Design review of the part built by this model. Coordinates are the model's own, in mm. A direction names the side the tool comes from. Give positions to 0.01 mm unless a question says otherwise; leave off trailing zeros. Order: outer loops, then holes, each group sorted by start corner. A loop starts at its lowest first (then second) coordinate and runs counter-clockwise, first axis right, second up. Notation, with made-up numbers: (44, 7.5) -> (63, 7.5) arc R19 ccw to (63, 19.5) -> close; hole circle Ø1 at (89.25, -9). An arc over 180 degrees is marked (long way). One line per item, written item: value. Start each with the question number.
1) Tool access review of faces 5 (the face through (6, 0, -5)), 6 (the face through (4.88, -1.08, -19.68)), 7 (the face through (2.6, -0.1, -11.4)): name each direction out of +Z, -Z, +X, -X, +Y, -Y from which nothing blocks a thin tool from reaching the whole face with its end or side.
2) Consider section C-C (x = 0). State the section outline as (y, z) points, plus the area to 3 significant figures.
3) Consider section B-B (z = 0). State the section outline as (x, y) points.
4) The part is to be moulded in two halves that separate along Z. For faces 1 (the face through (-4, -3, 0)), 2 (the face through (3, 1, -24)), 3 (the face through (5, -3, 0)), 4 (the face through (4, 6, -7)), say which applies: released by +Z, released by -Z, zero draft, split by the parting line, or undercut.
5) Wall thickness on line 1 along X through (y, z) = (4.25, -8.5); line 2 along X through (y, z) = (-0.25, 6); line 3 along Z through (x, y) = (5.35, 0): over which ranges is each line inside the solid? List them lowest first. Write a range as from..to.
6) Consider section D-D (z = -5). State the section outline as (x, y) points, plus the area to 3 significant figures.
7) Consider section A-A (y = 0). State how many separate pieces and enclosed holes the cut face has, plus the area to 3 significant figures.
8) For pin 1 (3.5 mm diameter, centred on y = 0, z = 0, fed in from +X); pin 2 (1 mm diameter, centred on x = -4.5, y = -3, fed in from +Z), all flat-tipped, find the tip position at first contact; note any pin that passes through.
from build123d import *

# Parameters (mm, degrees)
CUT_EXTRUDE1_DEPTH           = 13
CUT_EXTRUDE1_DEPTH_BACK      = 13
CUT_EXTRUDE2_DEPTH           = 13
CUT_EXTRUDE2_DEPTH_BACK      = 13
CUT_EXTRUDE3_DEPTH           = 13
CUT_EXTRUDE3_DEPTH_BACK      = 13
SKETCH5_W                    = 16.2
SKETCH5_H                    = 3
CUT_REVOLVE3_ANGLE           = 90
CUT_REVOLVE3_OTHER_WAY_ANGLE = 90


with BuildPart() as part:
    # Sketch1 → Revolve1 (revolve)
    with BuildSketch(Plane(origin=(0, 0, 0), x_dir=(0, 0, -1), z_dir=(1, 0, 0))):
        with BuildLine():
            Line((-7, 0), (-7, 12))
            Line((-7, 12), (13.325317547, 12))
            Line((13.325317547, 12), (15, 5.75))
            ThreePointArc((15, 5.75), (15.219669914, 5.219669914), (15.75, 5))
            Line((15.75, 5), (23.5, 5))
            ThreePointArc((23.5, 5), (23.853553391, 4.853553391), (24, 4.5))
            Line((24, 4.5), (24, 0))
            Line((24, 0), (-7, 0))
        make_face()
    revolve(axis=Axis((0, 0, -24), (0, 0, 1)))

    # Sketch2 → Cut-Extrude1 (cut, two sides)
    with BuildSketch(Plane(origin=(0, 0, 0), x_dir=(1, 0, 0), z_dir=(0, 1, 0))) as cut_extrude1_sk:
        Polygon((-3, 11), (-3, -8), (3, -8), (3, 11), (2, 12), (-2, 12), align=None)
    extrude(amount=CUT_EXTRUDE1_DEPTH, mode=Mode.SUBTRACT)
    extrude(cut_extrude1_sk.sketch, amount=-CUT_EXTRUDE1_DEPTH_BACK, mode=Mode.SUBTRACT)

    # Sketch3 → Cut-Extrude2 (cut, two sides)
    with BuildSketch(Plane(origin=(0, 0, 0), x_dir=(0, 0, -1), z_dir=(1, 0, 0))) as cut_extrude2_sk:
        Polygon((-20, -18), (24, -18), (24, -6), (-8, -6), (-8, 6), (24, 6), (24, 18), (-20, 18), align=None)
    extrude(amount=CUT_EXTRUDE2_DEPTH, mode=Mode.SUBTRACT)
    extrude(cut_extrude2_sk.sketch, amount=-CUT_EXTRUDE2_DEPTH_BACK, mode=Mode.SUBTRACT)

    # Sketch4 → Cut-Extrude3 (cut, two sides)
    with BuildSketch(Plane(origin=(0, 0, 0), x_dir=(1, 0, 0), z_dir=(0, 1, 0))) as cut_extrude3_sk:
        Polygon((-18, -20), (18, -20), (18, 24), (6, 24), (6, -8), (-6, -8), (-6, 24), (-18, 24), align=None)
    extrude(amount=CUT_EXTRUDE3_DEPTH, mode=Mode.SUBTRACT)
    extrude(cut_extrude3_sk.sketch, amount=-CUT_EXTRUDE3_DEPTH_BACK, mode=Mode.SUBTRACT)

    # Sketch5 → Cut-Revolve1 (revolve, cut)
    with BuildSketch(Plane.XY):
        with Locations((0, 1.5)):
            Rectangle(SKETCH5_W, SKETCH5_H)
    revolve(axis=Axis((8.1, 0, 0), (-1, 0, 0)), mode=Mode.SUBTRACT)

    # Sketch6 → Cut-Revolve2 (revolve, cut)
    with BuildSketch(Plane(origin=(0, 0, 0), x_dir=(0, 0, -1), z_dir=(1, 0, 0))):
        Polygon((10.9, 0), (10.9, 2.4585), (23.5585, 2.4585), (24.1, 3), (24.1, 0), align=None)
    revolve(axis=Axis((0, 0, -24.1), (0, 0, 1)), mode=Mode.SUBTRACT)

    # Sketch7 → Cut-Revolve3 (revolve, cut)
    with BuildSketch(Plane(origin=(0, 0, 0), x_dir=(1, 0, 0), z_dir=(0, 1, 0))):
        Polygon((-7, -18.589270357), (0, -22.630722241), (7, -18.589270357), (7, -4.732863896), (0, -8.774315781), (-7, -4.732863896), align=None)
    revolve(axis=Axis((-7, 0, -12), (1, 0, 0)), revolution_arc=CUT_REVOLVE3_ANGLE, mode=Mode.SUBTRACT)

    # Sketch7 → Cut-Revolve3 other way (revolve, cut)
    with BuildSketch(Plane(origin=(0, 0, 0), x_dir=(1, 0, 0), z_dir=(0, 1, 0))):
        Polygon((-7, -18.589270357), (0, -22.630722241), (7, -18.589270357), (7, -4.732863896), (0, -8.774315781), (-7, -4.732863896), align=None)
    revolve(axis=Axis((-7, 0, -12), (-1, 0, 0)), revolution_arc=CUT_REVOLVE3_OTHER_WAY_ANGLE, mode=Mode.SUBTRACT)


solid = part.part
Checked values:
1. face 5: +Z, -Z, +X, +Y, -Y
1. face 6: -Z
1. face 7: +Z, +Y, -Y
2. outline: (-6, -14.93) -> (-5.75, -15) arc R0.75 cw to (-5, -15.75) -> (-5, -23.5) arc R0.5 ccw to (-4.5, -24) -> (-2.9, -24) -> (-2.46, -23.56) -> (-2.46, -12) -> (-6, -12) -> close; (2.46, -23.56) -> (2.9, -24) -> (4.5, -24) arc R0.5 ccw to (5, -23.5) -> (5, -15.75) arc R0.75 cw to (5.75, -15) -> (6, -14.93) -> (6, -12) -> (2.46, -12) -> close
2. area: 66.9 mm^2
3. outline: (-6, -6) -> (-3, -6) -> (-3, -3) -> (-6, -3) -> close; (-6, 3) -> (-3, 3) -> (-3, 6) -> (-6, 6) -> close; (3, -6) -> (6, -6) -> (6, -3) -> (3, -3) -> close; (3, 3) -> (6, 3) -> (6, 6) -> (3, 6) -> close
4. face 1: undercut
4. face 2: released by -Z
4. face 3: undercut
4. face 4: zero draft
5. line 1: x = -6..-3, 3..6
5. line 2: x = -4.8..-3, 3..4.8
5. line 3: z = -15.12..-3, 3..5.69
6. outline: (-6, -6) -> (-3, -6) -> (-3, 6) -> (-6, 6) -> close; (3, -6) -> (6, -6) -> (6, 6) -> (3, 6) -> close
6. area: 72.0 mm^2
7. separate pieces: 4
7. enclosed holes: 0
7. area: 141 mm^2
8. pin 1: passes through
8. pin 2: stops at z = 6.23
